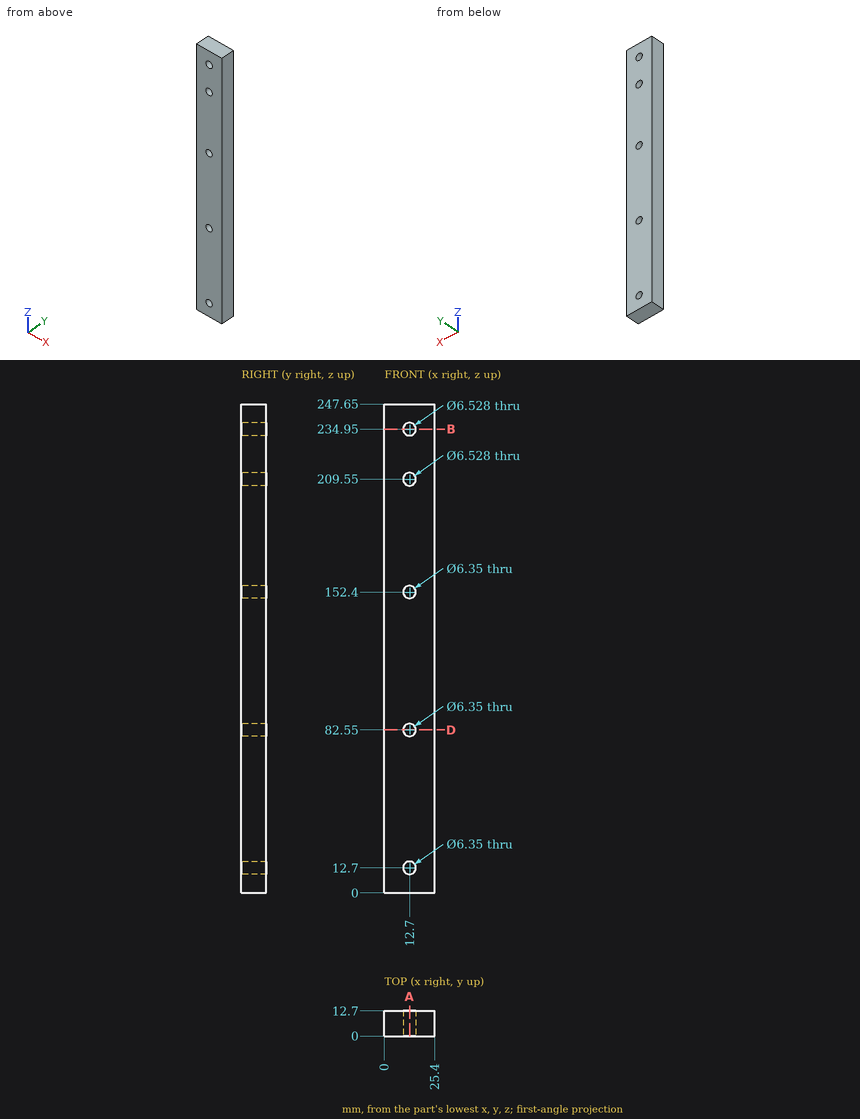
Here's the drawing with two shaded views (mm, measured from the low corner). I have some questions. Coordinates: 2 decimals unless noted, no trailing zeros. Write each loop counter-clockwise with the first axis right and the second up, starting at its lowest first coordinate (ties: lowest second). Pieces come first, ordered by that corner, then holes. Notation, with made-up numbers: (-25, -15.5) -> (8, -15.5) arc R34 cw to (8, 22.5) -> close; hole circle Ø2 at (6.5, 44.25). An arc over 180 degrees is marked (long way). Write item = value, one per line. Start each with the question number.
(1) Will this pin go through, and if not, where does the flat tip stop? pin 1 (6 mm diameter, centred on y = 2.5, z = 199.5, fed in from -X).
(2) I want a section at A-A (x = 12.7). Give the number of separate pieces and of enclosed holes in the cut face, plus the area to 3 significant figures.
(3) I want a section at B-B (z = 234.95). Please give me the cut outline in (x, y).
(4) I need wall thicknesses on line 1 (X direction, y = 10, z = 152.4) (3 decimals); line 2 (Z direction, x = 13.5, y = 8); line 3 (X direction, y = 7.5, z = 234.95). Which ranges of each line are inside material? Lowest first, please. Write a range as [from, to].
(5) I want a section at D-D (z = 82.55). Please give me the cut outline in (x, y) (3 decimals), plus the area to 3 significant figures.
Result set:
q1.pin_1 = 0
q2.separate_pieces = 6
q2.enclosed_holes = 0
q2.area = 2,740 mm2
q3.outline = (0, 0) -> (9.44, 0) -> (9.44, 12.7) -> (0, 12.7) -> close; (15.96, 0) -> (25.4, 0) -> (25.4, 12.7) -> (15.96, 12.7) -> close
q4.line_1 = [0, 9.525], [15.875, 25.4]
q4.line_2 = [0, 9.63], [15.77, 79.48], [85.62, 149.33], [155.47, 206.39], [212.71, 231.79], [238.11, 247.65]
q4.line_3 = [0, 9.44], [15.96, 25.4]
q5.outline = (0, 0) -> (9.525, 0) -> (9.525, 12.7) -> (0, 12.7) -> close; (15.875, 0) -> (25.4, 0) -> (25.4, 12.7) -> (15.875, 12.7) -> close
q5.area = 242 mm2
